Can you work these out from the model? Positions are in its coordinate system, mm. A direction names the side the tool comes from. Coordinates: 2 decimals unless noted, no trailing zeros. Order: outer loops, then holes, each group sorted by start corner. A loop starts at its lowest first (then second) coordinate and runs counter-clockwise, first axis right, second up. Notation, with made-up numbers: (54.5, 63) - (96.5, 63) arc R17 cw to (96.5, 93) - close; hole circle Ø8 at (56.25, 88). An arc over 180 degrees is marked (long way). Use a Markdown table: item, result. Add a question column.
(1) I want a section at D-D (z = -33.5). List the corners of the cut face in (x, y) for me.
(2) I want a section at B-B (x = -8). List the corners of the cut face in (y, z) for me, and give its area (3 significant figures).
(3) I want a section at A-A (z = -8.5). List the corners of the cut face in (x, y) for me.
(4) On a 3-axis mill with a long thin cutter (end or side, diameter ignored), from which of +Z, -Z, +X, -X, +Y, -Y can I reach the whole of each face in a straight line? I mean faces 4 (the flat face through (-30, -25.4, 48)), 5 (the cylindrical face through (38.56, -12.52, 15.26)), 6 (the flat face through (63.269, -13, 5)). Say none if no direction works.
(5) If I drill on L1, parallel to Z at x = 0, y = -52; L2, parallel to Y at x = 50, z = 40.5; L3, parallel to Z at x = 0, y = -9, over which ranges is the centre line in solid material (lowest first)? Write a range as [from, to].
(6) I want a section at C-C (y = -5). List the corners of the cut face in (x, z) for me, and give its area (3 significant figures).
(7) We'd pull the mould along X, two halves only. Please class faces 1 (the cylindrical face through (-6.719, -50.444, 54.287)), 2 (the flat face through (-0.2, -25.4, 36.2)), 3 (the flat face through (-30, 0, 34)): pulls with the +X half, pulls with the -X half, needs draft (parallel to the pull), parting line crosses it, or undercut.
(8) For pin 1 Ø10 at (y, z) = (-38.5, -19.5) entering from +X; pin 2 Ø10 at (y, z) = (-65, 15.5) entering from +X; pin 3 Ø3 at (y, z) = (-48, 13) entering from +X, each with a flat end and sliding along its axis, tell me the tip position at first contact or that it passes through.
```python
from build123d import *

# Parameters (mm, degrees)
F1_R     = 40.425581
F2_DEPTH = 25.4
F3_R     = 51.609341
F4_DEPTH = 50.8
F5_R     = 32.796001
F6_DEPTH = 76.2


with BuildPart() as f2:
    # F1 (on face) → F2 (new body)
    with BuildSketch(Plane.XZ):
        Polygon((63.269094, -55.995453), (63.269094, 67.540914), (-64.885452, 67.540914), (-64.885452, 55.995453), (-64.885452, -54.840911), align=None)
        with Locations((0, 3.117273)):
            Circle(F1_R, mode=Mode.SUBTRACT)
    extrude(amount=F2_DEPTH)

    # F3 (on face) → F4 (join)
    with BuildSketch(Plane.XZ.offset(25.4)):
        with Locations((0, 3.117273)):
            Circle(F3_R)
    extrude(amount=F4_DEPTH)

    # F5 (on face) → F6 (cut)
    with BuildSketch(Plane.XZ.offset(76.2)):
        with Locations((0, 3.117273)):
            Circle(F5_R)
    extrude(amount=-F6_DEPTH, mode=Mode.SUBTRACT)


solid = f2.part
```
Answers follow:
| question | item | result |
|---|---|---|
| 1 | outline | (-64.89, -25.4) - (-36.37, -25.4) - (-36.37, -76.2) - (36.37, -76.2) - (36.37, -25.4) - (63.27, -25.4) - (63.27, 0) - (17.13, 0) - (17.13, -25.4) - (-17.13, -25.4) - (-17.13, 0) - (-64.89, 0) - close |
| 2 | outline | (-76.2, -47.87) - (-25.4, -47.87) - (-25.4, -55.35) - (0, -55.35) - (0, -36.51) - (-25.4, -36.51) - (-25.4, -28.69) - (-76.2, -28.69) - close; (-76.2, 34.92) - (-25.4, 34.92) - (-25.4, 42.74) - (0, 42.74) - (0, 67.54) - (-25.4, 67.54) - (-25.4, 54.1) - (-76.2, 54.1) - close |
| 2 | area | 3,060 mm² |
| 3 | outline | (-64.89, -25.4) - (-50.28, -25.4) - (-50.28, -76.2) - (-30.67, -76.2) - (-30.67, -25.4) - (-38.72, -25.4) - (-38.72, 0) - (-64.89, 0) - close; (30.67, -76.2) - (50.28, -76.2) - (50.28, -25.4) - (63.27, -25.4) - (63.27, 0) - (38.72, 0) - (38.72, -25.4) - (30.67, -25.4) - close |
| 4 | face 4 | -Y |
| 4 | face 5 | +Y |
| 4 | face 6 | +Z, -Z, +X, +Y, -Y |
| 5 | L1 | z = [-48.49, -29.68], [35.91, 54.73] |
| 5 | L2 | y = [-25.4, 0] |
| 5 | L3 | z = [-55.43, -37.31], [43.54, 67.54] |
| 6 | outline | (-64.89, -54.84) - (63.27, -56) - (63.27, 67.54) - (-64.89, 67.54) - close; hole circle Ø80.85 at (0, 3.12) |
| 6 | area | 10,600 mm² |
| 7 | face 1 | parting line crosses it |
| 7 | face 2 | undercut |
| 7 | face 3 | needs draft |
| 8 | pin 1 | stops at x = 48.51 |
| 8 | pin 2 | stops at x = 51.08 |
| 8 | pin 3 | stops at x = 50.92 |
